Geometry: see drawing. Coordinates: mm, zero at the bounding-box minimum. A direction names the side the tool comes from. Give positions to 0.01 mm unless a question says otherwise; leave off trailing zeros. Order: outer loops, then holes, each group sorted by start corner. A loop starts at its lowest first (then second) coordinate and runs counter-clockwise, first axis right, second up. Notation, with made-up numbers: (-23.5, 15) - (9.5, 15) arc R23 cw to (9.5, 51) - close; hole circle Ø6 at (23, 47). An arc over 180 degrees is marked (long way). Put each result on its own line as item: value. Start each with the question number.
1. Section C-C on y = 3.5. Count the separate pieces of the cut face and the enclosed holes in it, plus the area to 3 significant figures.
2. Section A-A on z = 12.65. Return the cut outline in (x, y).
3. First-contact query: P1, Ø2, axis at x = 13, y = 3.5, coming from the +Z side; P2, Ø1.1, axis at y = 4.5, z = 51.5, coming from the -X side; P3, Ø1.8, axis at y = 3, z = 51.5, coming from the +X side. Flat tips, straight axial feed; report the tip coordinate or a pass-through.
4. Section B-B on x = 73.5. Return the cut outline in (y, z).
5. Ray query, line 1 along X through (y, z) = (5, 31.15); line 2 along Z through (x, y) = (35, 0.75); line 3 along X through (y, z) = (1.25, 30.5) (1 decimal). Return the intervals inside material, ascending. Write a range as from..to.
6. Mould query, pull axis Z, two halves, no side actions, for the marked faces 1, 2 and 3. Classes: pulls with the +Z half, pulls with the -Z half, needs draft (parallel to the pull), parting line crosses it, or undercut.
7. Set-up query: the marked faces 4 and 5. Return all of +Z, -Z, +X, -X, +Y, -Y with unobstructed straight access to the full face (end or side cutting, diameter ignored); none if empty.
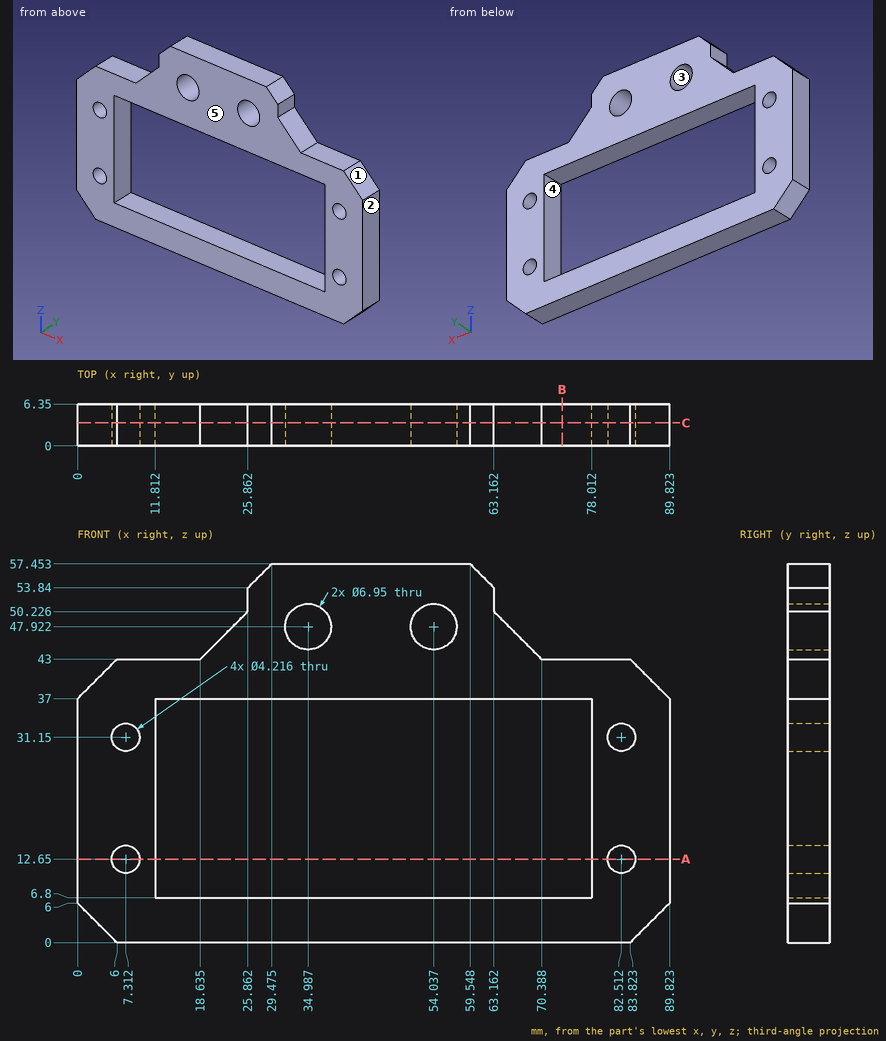
Resolved:
1. separate pieces: 1
1. enclosed holes: 7
1. area: 2,240 mm^2
2. outline: (0, 0) - (5.2, 0) - (5.2, 6.35) - (0, 6.35) - close; (9.42, 0) - (11.81, 0) - (11.81, 6.35) - (9.42, 6.35) - close; (78.01, 0) - (80.4, 0) - (80.4, 6.35) - (78.01, 6.35) - close; (84.62, 0) - (89.82, 0) - (89.82, 6.35) - (84.62, 6.35) - close
3. P1: z = 43
3. P2: x = 25.86
3. P3: x = 63.16
4. outline: (0, 0) - (6.35, 0) - (6.35, 6.8) - (0, 6.8) - close; (0, 37) - (6.35, 37) - (6.35, 43) - (0, 43) - close
5. line 1: 0..5.2, 9.42..11.81, 78.01..80.4, 84.62..89.82
5. line 2: 0..6.8, 37..44.45, 51.4..57.45
5. line 3: 0..5.3, 9.3..11.8, 78..80.5, 84.5..89.8
6. face 1: pulls with the +Z half
6. face 2: needs draft
6. face 3: undercut
7. face 4: +Y, -Y
7. face 5: +Z, -Z, +X, -X, -Y
